Can you work these out from the model? Positions are in its coordinate system, mm. A direction names the side the tool comes from. Give positions to 0.01 mm unless a question says otherwise; leave off trailing zeros. Loops run counter-clockwise (first coordinate to the right, second up) from the corner with the lowest first, then second, coordinate; pieces in that order, holes last. Notation, with made-up numbers: (52.25, -11.5) -> (93.25, -11.5) arc R11 cw to (93.25, 5.5) -> close; hole circle Ø10 at (64.5, 10.25). An arc over 180 degrees is marked (long way). One line per question, with ' | ' between items.
Autodesk Inventor part; units mm, degrees
ref_plane "YZ Plane" through (0, 0, 0) normal (1, 0, 0) x (0, 1, 0)
ref_plane "XZ Plane" through (0, 0, 0) normal (0, 1, 0) x (-1, 0, 0)
ref_plane "XY Plane" through (0, 0, 0) normal (0, 0, 1) x (1, 0, 0)
sketch "Sketch1" plane through (0, 0, 0) normal (0, 0, 1) x (1, 0, 0)
  line L0 (-17.78, 0) -> (17.78, 0)
  line L1 (0, -17.78) -> (0, 17.78)
  line L2 (-12.7, 12.7) -> (-12.7, -12.7)
  line L3 (-12.7, -12.7) -> (12.7, -12.7)
  line L4 (12.7, -9.525) -> (-9.525, -9.525)
  line L5 (-9.525, -9.525) -> (-9.525, 12.7)
  line L6 (-12.7, 12.7) -> (-9.525, 12.7)
  line L7 (12.7, -12.7) -> (12.7, -9.525)
  point P0 (0, 0)
  point P1 (-12.7, 0)
  point P2 (0, -12.7)
  dimension "d0" = 25.4
  dimension "d1" = 3.175
extrude "Extrusion1" add sketch "Sketch1" along normal mid plane 101.6 contours L2 L6 L5 L0 | L0 L5 L4 L1 L3 L2 | L1 L4 L7 L3
sketch "Sketch2" plane through (-9.525, -9.525, 50.8) normal (1, 0, 0) x (0, 0, -1)
  line L0 (0, 22.225) -> (0, 0)
  point P0 (50.8, 9.525)
  point P1 (25.4, 9.525)
  point P2 (76.2, 9.525)
  dimension "d4" = 50.8
  dimension "d5" = 25.4
hole "Hole1" at (-9.525, 0, 25.4) at (-9.525, 0, -25.4) direction (-1, 0, 0) diameter 6.7564 end through all
properties part number "angle template al-6061 1x1x0.125" material "Aluminum-6061"
Q1. On a 3-axis mill with a long thin cutter (end or side, diameter ignored), from which of +Z, -Z, +X, -X, +Y, -Y can I reach the whole of each face in a straight line? I mean faces 1 (the face through (0, -12.7, -1)), 2 (the face through (2, -9.525, -1)). Say none if no direction works.
Entries:
face 1: +Z, -Z, +X, -X, -Y | face 2: +Z, -Z, +X, +Y
Q2. If I drill on probe 1 along Z at (x, y) = (-10.4, 0); probe 2 along Y at (x, z) = (-11.25, 25.4); probe 3 along X at (y, z) = (9, 0.5) (3 decimals), over which ranges is the centre line in solid material (lowest first)? Write a range as from..to.
Entries:
probe 1: -50.8..-28.78, -22.02..22.02, 28.78..50.8 | probe 2: -12.7..-3.38, 3.38..12.7 | probe 3: -12.7..-9.525
Q3. If we section it at B-B (y = 0): Write out the boundary of the cut face in (x, z) (3 decimals).
Entries:
outline: (-12.7, -50.8) -> (-9.525, -50.8) -> (-9.525, -28.778) -> (-12.7, -28.778) -> close; (-12.7, -22.022) -> (-9.525, -22.022) -> (-9.525, 22.022) -> (-12.7, 22.022) -> close; (-12.7, 28.778) -> (-9.525, 28.778) -> (-9.525, 50.8) -> (-12.7, 50.8) -> close
Q4. If we section it at C-C (y = 9.25): Write out the boundary of the cut face in (x, z) (3 decimals), plus the area to 3 significant figures.
Entries:
outline: (-12.7, -50.8) -> (-9.525, -50.8) -> (-9.525, 50.8) -> (-12.7, 50.8) -> close | area: 323 mm²
Q5. If we mould it in two halves opening along Z, with no side actions, what happens to faces 3 (the face through (-11.135, -0.149, 28.775)), 4 (the face through (-9.525, 1, -1)), 5 (the face through (-6, -10, -50.8))? For each: pulls with the +Z half, pulls with the -Z half, needs draft (parallel to the pull), parting line crosses it, or undercut.
Entries:
face 3: undercut | face 4: needs draft | face 5: pulls with the -Z half
Q6. For pin 1 Ø5.5 at (y, z) = (0, 25.4) entering from +X; pin 2 Ø2 at (y, z) = (-2.5, 1.5) entering from +X (3 decimals); pin 3 Ø12 at (x, z) = (4, -19.5) entering from +Y (3 decimals), each with a flat end and sliding along its axis, tell me the tip position at first contact or that it passes through.
Entries:
pin 1: through | pin 2: x = -9.525 | pin 3: y = -9.525
Q7. If we section it at A-A (z = 25.4): Write out the boundary of the cut face in (x, y) (3 decimals).
Entries:
outline: (-12.7, -12.7) -> (12.7, -12.7) -> (12.7, -9.525) -> (-9.525, -9.525) -> (-9.525, -3.378) -> (-12.7, -3.378) -> close; (-12.7, 3.378) -> (-9.525, 3.378) -> (-9.525, 12.7) -> (-12.7, 12.7) -> close
